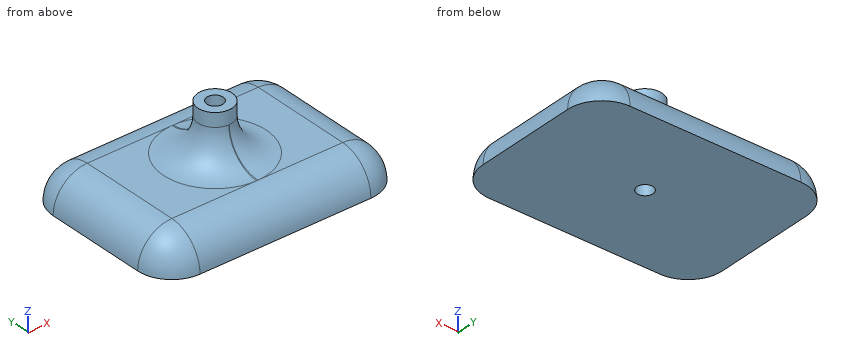
```python
from build123d import *

# Parameters (mm, degrees)
ESBO_O1_W                = 70
ESBO_O1_H                = 50
ESBO_O1_R                = 2.35
RESSALTO_EXTRUS_O1_DEPTH = 10
ESBO_O2_R                = 5.001389376
ESBO_O2_R_2              = 2.35
RESSALTO_EXTRUS_O2_DEPTH = 24
FILETE1_R                = 10
FILETE2_R                = 10
FILETE3_R                = 10
FILETE4_R                = 10
FILETE5_R                = 10


with BuildPart() as part:
    # Esboço1 → Ressalto-extrusão1 (new body)
    with BuildSketch(Plane.XY):
        with Locations((-0.869381548, 25)):
            Rectangle(ESBO_O1_W, ESBO_O1_H)
        with Locations((-0.869381548, 25)):
            Circle(ESBO_O1_R, mode=Mode.SUBTRACT)
    extrude(amount=RESSALTO_EXTRUS_O1_DEPTH)

    # Esboço2 → Ressalto-extrusão2 (add)
    with BuildSketch(Plane.XY):
        with Locations(Location((-0.869381548, 25, 0), (0, 0, 180))):
            Circle(ESBO_O2_R)
        with Locations((-0.869381548, 25)):
            Circle(ESBO_O2_R_2, mode=Mode.SUBTRACT)
    extrude(amount=RESSALTO_EXTRUS_O2_DEPTH)

    # Filete1
    filete1_edges = [part.edges().sort_by_distance(p)[0] for p in [
        (-0.869381548, 0, 10),
    ]]
    fillet(filete1_edges, radius=FILETE1_R - 0.0001)  # a hair under: the kernel refuses the full size

    # Filete2
    filete2_edges = [part.edges().sort_by_distance(p)[0] for p in [
        (-0.869381548, 50, 10),
    ]]
    fillet(filete2_edges, radius=FILETE2_R - 0.0001)  # a hair under: the kernel refuses the full size

    # Filete3
    filete3_edges = [part.edges().sort_by_distance(p)[0] for p in [
        (-35.869381548, 2.928902899, 7.071097101),
        (-35.869381548, 25, 10),
        (-35.869381548, 47.071097101, 7.071097101),
    ]]
    fillet(filete3_edges, radius=FILETE3_R - 0.0001)  # a hair under: the kernel refuses the full size

    # Filete4
    filete4_edges = [part.edges().sort_by_distance(p)[0] for p in [
        (34.130618452, 25, 10),
        (34.130618452, 2.928902899, 7.071097101),
        (34.130618452, 47.071097101, 7.071097101),
    ]]
    fillet(filete4_edges, radius=FILETE4_R - 0.0001)  # a hair under: the kernel refuses the full size

    # Filete5
    filete5_edges = [part.edges().sort_by_distance(p)[0] for p in [
        (4.132007829, 25, 10),
    ]]
    fillet(filete5_edges, radius=FILETE5_R)


solid = part.part
```
For this review, take the finished solid that the model builds, in its own axes (mm). Coordinates: 2 decimals unless noted, no trailing zeros. Write each loop counter-clockwise with the first axis right and the second up, starting at its lowest first coordinate (ties: lowest second). Pieces come first, ordered by that corner, then holes. Notation, with made-up numbers: (19, -31.5) - (33, -31.5) arc R27 cw to (33, -9.5) - close; hole circle Ø7 at (84.25, 8). An arc over 180 degrees is marked (long way). Put each result on its own line as item: value.
1. Add section D-D, the plane z = 21. Give the boundary of the cut face in (x, y), then the cut area to 3 significant figures.
Values found:
outline: circle Ø10 at (-0.87, 25); hole circle Ø4.7 at (-0.87, 25)
area: 61.2 mm²
2. For pin 1 (7.5 mm diameter, centred on x = -0.87, y = 25, fed in from -Z); pin 2 (2 mm diameter, centred on x = 19, z = 9.5, fed in from +Y); pin 3 (10 mm diameter, centred on y = 7.5, z = 7.5, fed in from +X); pin 4 (4 mm diameter, centred on x = 25, z = 9, fed in from -Y), all flat-tipped, find the tip position at first contact; note any pin that passes through.
Values found:
pin 1: z = 0
pin 2: y = 45.27
pin 3: x = 33.7
pin 4: y = 2.9
3. Wall thickness on probe 1 along X at (y, z) = (27, 18.5); probe 2 along Z at (x, y) = (-21, 23); probe 3 along Y at (x, z) = (-2, 16): over which ranges is each line inside the solid? List them lowest first.
Values found:
probe 1: -5.58 to -2.1, 0.36 to 3.84
probe 2: 0 to 10
probe 3: 19.27 to 22.94, 27.06 to 30.73
4. Add section B-B, the plane z = 7.75. Give the boundary of the cut face in (x, y), then the cut area to 3 significant figures.
Values found:
outline: (-32.19, 10) arc R6.32 ccw to (-25.87, 3.68) - (24.13, 3.68) arc R6.32 ccw to (30.45, 10) - (30.45, 40) arc R6.32 ccw to (24.13, 46.32) - (-25.87, 46.32) arc R6.32 ccw to (-32.19, 40) - close; hole circle Ø4.7 at (-0.87, 25)
area: 2,620 mm²
